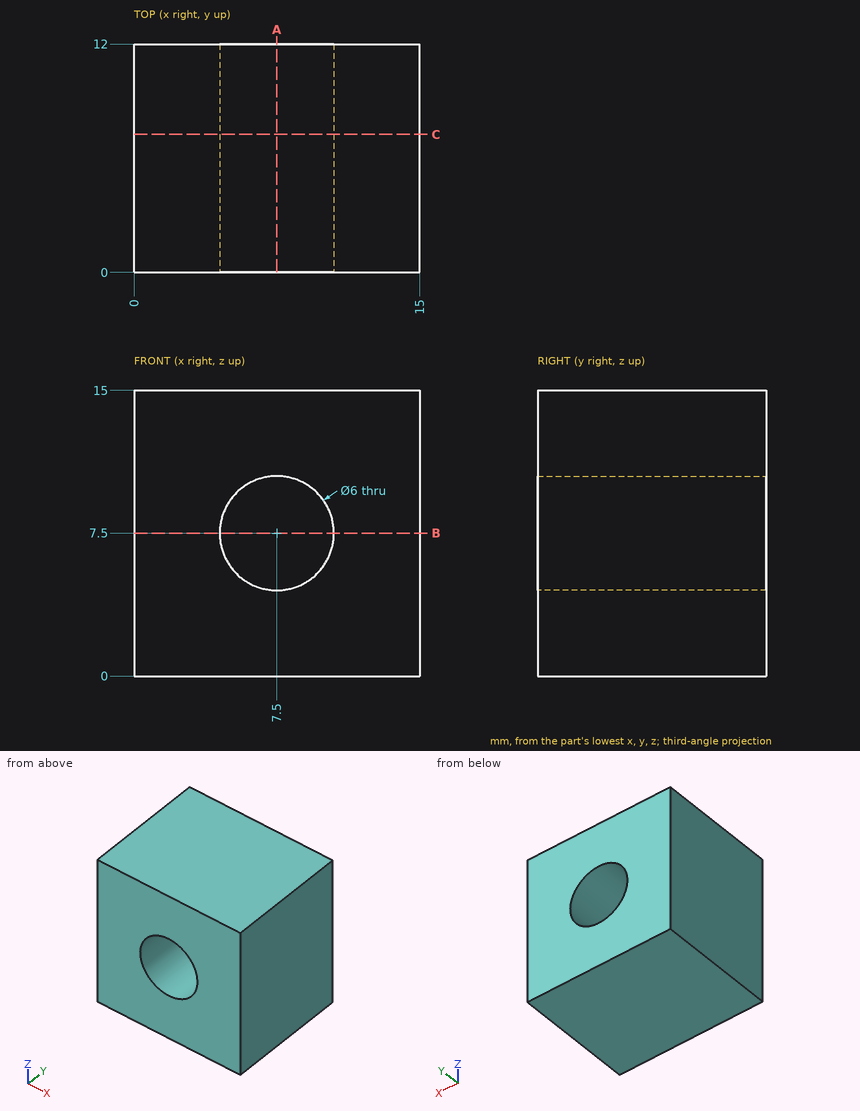
Check sheet for the drawn part. Datum: minimum x, y, z corner. Units: mm. Give positions to 0.01 mm unless a question says otherwise; leave off trailing zeros. Order: outer loops, then holes, each group sorted by start corner. A loop starts at its lowest first (then second) coordinate and runs counter-clockwise, first axis right, second up. Notation, with made-up numbers: (52, 56) - (103, 56) arc R10 cw to (103, 61) - close; hole circle Ø5 at (55.5, 20.25). An arc over 180 degrees is marked (long way). Answer in a Markdown table with one row per item. Add a question column.
Q1. Cross-section at A-A, the plane x = 7.5. Enter the section's corners in (y, z).
Q2. Material ranges on probe 1 along Z at (x, y) = (7.5, 9.25); probe 2 along Z at (x, y) = (5, 8.75), recorded low to high. Write a range as from..to.
Q3. Cross-section at B-B, the plane z = 7.5. Enter the section's corners in (x, y), then the cut area to 3 significant figures.
Q4. Gauge pin test, flat end, axial feed: pin 1 (4 mm diameter, centred on x = 2, z = 10.5, fed in from -Y). Record the tip position at first contact, or that the pin passes through.
Q5. Cross-section at C-C, the plane y = 7.25. Enter the section's corners in (x, z), then the cut area to 3 significant figures.
Check values:
| question | item | result |
|---|---|---|
| 1 | outline | (0, 0) - (12, 0) - (12, 4.5) - (0, 4.5) - close; (0, 10.5) - (12, 10.5) - (12, 15) - (0, 15) - close |
| 2 | probe 1 | z = 0..4.5, 10.5..15 |
| 2 | probe 2 | z = 0..5.84, 9.16..15 |
| 3 | outline | (0, 0) - (4.5, 0) - (4.5, 12) - (0, 12) - close; (10.5, 0) - (15, 0) - (15, 12) - (10.5, 12) - close |
| 3 | area | 108 mm^2 |
| 4 | pin 1 | stops at y = 0 |
| 5 | outline | (0, 0) - (15, 0) - (15, 15) - (0, 15) - close; hole circle Ø6 at (7.5, 7.5) |
| 5 | area | 197 mm^2 |
